Can you work these out from the model? Positions are in its coordinate system, mm. Face numbers are marked on the shaded views. A direction names the side the tool comes from. Give positions to 0.01 mm unless a question says otherwise; leave off trailing zeros. Loops run counter-clockwise (first coordinate to the right, second up) from the corner with the lowest first, then second, coordinate; pieces in that order, holes last. Notation, with made-up numbers: (-17.5, -9) -> (27.5, -9) arc R31 ccw to (27.5, 18) -> close; hole circle Ø4 at (-29.5, -35). An arc over 180 degrees is marked (long way). Use CSV: the item, a comma, the result in double quotes.
from build123d import *

# Parameters (mm, degrees)
SKETCH1_W           = 20
SKETCH1_H           = 20
BOSS_EXTRUDE1_DEPTH = 70
BOSS_EXTRUDE1_TAPER = 5
SKETCH2_R           = 2
CUT_EXTRUDE1_DEPTH  = 12.5
SKETCH3_W           = 55
SKETCH3_H           = 55
BOSS_EXTRUDE2_DEPTH = 3
FILLET1_R           = 4
SKETCH5_R           = 2.5
CUT_EXTRUDE2_DEPTH  = 10


with BuildPart() as part:
    # Sketch1 → Boss-Extrude1 (new body)
    with BuildSketch(Plane(origin=(0, 0, 0), x_dir=(1, 0, 0), z_dir=(0, 1, 0))):
        Rectangle(SKETCH1_W, SKETCH1_H)
    extrude(amount=BOSS_EXTRUDE1_DEPTH, taper=BOSS_EXTRUDE1_TAPER)

    # Sketch2 → Cut-Extrude1 (cut)
    with BuildSketch(Plane(origin=(0, 70, 0), x_dir=(1, 0, 0), z_dir=(0, 1, 0))):
        with Locations(Location((0, 0, 0), (0, 0, 270))):
            Circle(SKETCH2_R)
    extrude(amount=-CUT_EXTRUDE1_DEPTH, mode=Mode.SUBTRACT)

    # Sketch3 → Boss-Extrude2 (add)
    with BuildSketch(Plane.XZ):
        Rectangle(SKETCH3_W, SKETCH3_H)
    extrude(amount=-BOSS_EXTRUDE2_DEPTH)

    # Fillet1
    fillet1_edges = [part.edges().sort_by_distance(p)[0] for p in [
        (0, 3, 9.737534009),
        (0, 3, -9.737534009),
        (9.737534009, 3, 0),
        (-9.737534009, 3, 0),
    ]]
    fillet(fillet1_edges, radius=FILLET1_R)

    # Sketch5 → Cut-Extrude2 (cut)
    with BuildSketch(Plane(origin=(0, 3, 0), x_dir=(1, 0, 0), z_dir=(0, 1, 0))):
        with Locations(Location((-20, 0, 0), (0, 0, 270))):
            Circle(SKETCH5_R)
        with Locations(Location((0, 20, 0), (0, 0, 270))):
            Circle(SKETCH5_R)
        with Locations(Location((20, 0, 0), (0, 0, 270))):
            Circle(SKETCH5_R)
        with Locations(Location((0, -20, 0), (0, 0, 270))):
            Circle(SKETCH5_R)
    extrude(amount=-CUT_EXTRUDE2_DEPTH, mode=Mode.SUBTRACT)


solid = part.part
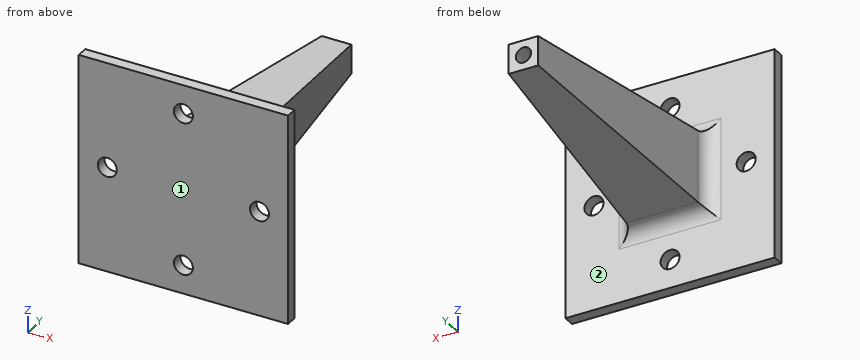
(1) If we section it at B-B, the plane x = 20: Write out the boundary of the cut face in (y, z), then the cut area to 3 significant figures.
Answer sheet:
outline,"(0, -27.5) -> (3, -27.5) -> (3, -2.5) -> (0, -2.5) -> close; (0, 2.5) -> (3, 2.5) -> (3, 27.5) -> (0, 27.5) -> close"
area,"150 mm2"
(2) If we section it at C-C, the plane z = 0: Give the number of separate pieces and of enclosed holes in the cut face, then the cut area to 3 significant figures.
Answer sheet:
separate pieces,"3"
enclosed holes,"0"
area,"1,000 mm2"
(3) If we section it at A-A, the plane z = -18.5: Write out the boundary of the cut face in (x, y).
Answer sheet:
outline,"(-27.5, 0) -> (-2, 0) -> (-2, 3) -> (-27.5, 3) -> close; (2, 0) -> (27.5, 0) -> (27.5, 3) -> (2, 3) -> close"
(4) Which directions (+Z, -Z, +X, -X, +Y, -Y) give clear straight access to the entire face, cutting with the end or side of a thin tool? Please do the marked faces 1 and 2.
Answer sheet:
face 1,"+Z, -Z, +X, -X, -Y"
face 2,"+Y"
(5) If I drill on L1, parallel to X at y = 2.35, z = 0; L2, parallel to X at y = 1, z = 20; L3, parallel to Y at x = 17.5, z = -4, over which ranges is the centre line in solid material (lowest first)? Write a range as from..to.
Answer sheet:
L1,"x = -27.5..-22.5, -17.5..17.5, 22.5..27.5"
L2,"x = -27.5..-2.5, 2.5..27.5"
L3,"y = 0..3"
(6) Will these pins go through, and if not, where does the flat tip stop? pin 1 Ø8 at (x, z) = (0, -20) entering from +Y; pin 2 Ø5 at (y, z) = (60, -7) entering from +X; pin 3 Ø6 at (y, z) = (26.5, 5.5) entering from +X; pin 4 Ø3 at (x, z) = (20, 0) entering from +Y.
Answer sheet:
pin 1,"stops at y = 3"
pin 2,"stops at x = 4.86"
pin 3,"stops at x = 7.94"
pin 4,"passes through"
